Read the model definition and answer for the solid it produces. Units are mm, in the model's axes. Face numbers are marked on the shaded views. Coordinates: 2 decimals unless noted, no trailing zeros. Order: outer loops, then holes, each group sorted by start corner. A loop starts at its lowest first (then second) coordinate and runs counter-clockwise, first axis right, second up. Notation, with made-up numbers: (15.5, 26.5) -> (47.5, 26.5) arc R20 ccw to (47.5, 55.5) -> close; hole circle Ø6 at (-29, 32). An arc over 180 degrees is marked (long way). Answer as a JSON object with one key per item and string values. Group by question number.
1) Determine the mould class of the marked faces 1, 2 and 3 for opening direction Y: released by +Y, released by -Y, zero draft, split by the parting line, or undercut.
2) Section D-D on x = 6 is taken. Determine the outline of the cut face in (y, z), and give its area (3 significant figures).
3) Consider L1, parallel to X at y = -0.75, z = 101.6; L2, parallel to Y at x = 13, z = 32.5; L3, parallel to Y at x = 27.5, z = 86.5. Determine where each line is inside the solid, lowest interval first.
4) Section C-C on z = 85 is taken. Determine the outline of the cut face in (x, y) (3 decimals), and give its area (3 significant figures).
5) Section A-A on x = 29 is taken. Determine the outline of the cut face in (y, z).
6) Given pin 1 (2 mm diameter, centred on y = -16, z = 58.5, fed in from +X); pin 2 (12 mm diameter, centred on x = 17, z = 80.5, fed in from -Y); pin 3 (3 mm diameter, centred on y = -11.5, z = 48, fed in from +X), each flat-ended and moving along its own axis, determine where each tip first touches the part or whether it passes through.
7) Section B-B on z = 101.6 is taken. Determine the outline of the cut face in (x, y) (3 decimals), and give its area (3 significant figures).
from build123d import *

# Parameters (mm, degrees)
BASE_FLANGE1_DEPTH = 127
CUT_EXTRUDE1_REACH = 146.789
SKETCH6_R          = 3.175
CUT_EXTRUDE2_REACH = 139.304
SKETCH7_R          = 3.175


# Read off the part's stored shape, not the designer's step: Base-Flange1
with BuildPart() as part:
    # Base-Flange1 outline → Base-Flange1 (new body)
    with BuildSketch(Plane.XY):
        with BuildLine():
            Line((44.523372088, -7.173652981), (24.703656185, -49.677170897))
            Line((24.703656185, -49.677170897), (27.111570966, -50.8))
            Line((27.111570966, -50.8), (46.931286869, -8.296482084))
            ThreePointArc((46.931286869, -8.296482084), (46.564368833, -2.698394652), (41.645844864, 0))
            Line((41.645844864, 0), (0, 0))
            Line((0, 0), (0, -2.65684))
            Line((0, -2.65684), (41.645844864, -2.65684))
            ThreePointArc((41.645844864, -2.65684), (44.323612704, -4.125913744), (44.523372088, -7.173652981))
        make_face()
    extrude(amount=BASE_FLANGE1_DEPTH)

    # Sketch6 → Cut-Extrude1 (cut, up to next)
    with BuildSketch(Plane(origin=(0, 0, 0), x_dir=(1, 0, 0), z_dir=(0, 1, 0)), mode=Mode.PRIVATE) as cut_extrude1_sk1:
        with Locations(Location((16.245844864, -101.6, 0), (0, 0, 270))):
            Circle(SKETCH6_R)
    cut_extrude1_tool1 = extrude(cut_extrude1_sk1.sketch, amount=-CUT_EXTRUDE1_REACH, mode=Mode.PRIVATE) & part.part
    # Sketch6 → Cut-Extrude1 (cut, up to next)
    with BuildSketch(Plane(origin=(0, 0, 0), x_dir=(1, 0, 0), z_dir=(0, 1, 0)), mode=Mode.PRIVATE) as cut_extrude1_sk2:
        with Locations(Location((16.245844864, -25.4, 0), (0, 0, 270))):
            Circle(SKETCH6_R)
    cut_extrude1_tool2 = extrude(cut_extrude1_sk2.sketch, amount=-CUT_EXTRUDE1_REACH, mode=Mode.PRIVATE) & part.part
    add(cut_extrude1_tool1.solids().sort_by_distance((16.245845, 0, 101.6))[0], mode=Mode.SUBTRACT)
    add(cut_extrude1_tool2.solids().sort_by_distance((16.245845, 0, 25.4))[0], mode=Mode.SUBTRACT)

    # Sketch7 → Cut-Extrude2 (cut, up to next)
    with BuildSketch(Plane(origin=(41.726805286, -19.457528855, 0), x_dir=(0, 0, -1), z_dir=(0.906307787036648, -0.4226182617407038, 0)), mode=Mode.PRIVATE) as cut_extrude2_sk1:
        with Locations(Location((-101.6, -12.580218597, 0), (0, 0, 90))):
            Circle(SKETCH7_R)
    cut_extrude2_tool1 = extrude(cut_extrude2_sk1.sketch, amount=-CUT_EXTRUDE2_REACH, mode=Mode.PRIVATE) & part.part
    # Sketch7 → Cut-Extrude2 (cut, up to next)
    with BuildSketch(Plane(origin=(41.726805286, -19.457528855, 0), x_dir=(0, 0, -1), z_dir=(0.906307787036648, -0.4226182617407038, 0)), mode=Mode.PRIVATE) as cut_extrude2_sk2:
        with Locations(Location((-25.4, -12.580218597, 0), (0, 0, 90))):
            Circle(SKETCH7_R)
    cut_extrude2_tool2 = extrude(cut_extrude2_sk2.sketch, amount=-CUT_EXTRUDE2_REACH, mode=Mode.PRIVATE) & part.part
    add(cut_extrude2_tool1.solids().sort_by_distance((36.410175, -30.859079, 101.6))[0], mode=Mode.SUBTRACT)
    add(cut_extrude2_tool2.solids().sort_by_distance((36.410175, -30.859079, 25.4))[0], mode=Mode.SUBTRACT)


solid = part.part
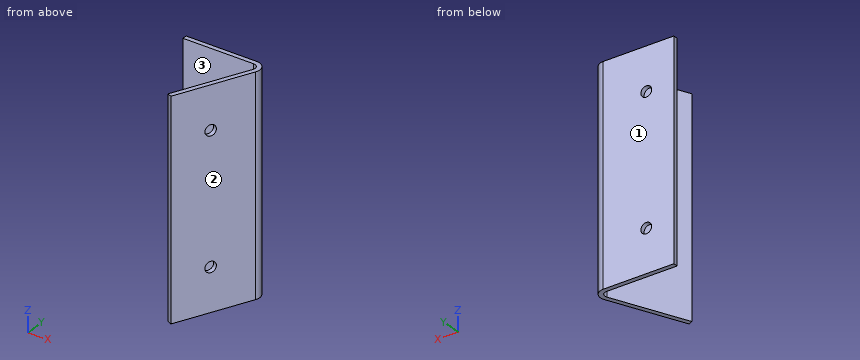
Worked answers:
{
 "1": {"face 1": "released by +Y", "face 2": "released by -Y", "face 3": "undercut"},
 "2": {"outline": "(-2.66, 0) -> (0, 0) -> (0, 127) -> (-2.66, 127) -> close", "area": "337 mm²"},
 "3": {"L1": "x = 0 to 13.07, 19.42 to 44.51", "L2": "y = -2.66 to 0", "L3": "y = -49.97 to -43.68, -2.66 to 0"},
 "4": {"outline": "(0, -2.657) -> (41.646, -2.657) arc R3.175 cw to (44.523, -7.174) -> (24.704, -49.677) -> (27.112, -50.8) -> (46.931, -8.296) arc R5.832 ccw to (41.646, 0) -> (0, 0) -> close", "area": "259 mm²"},
 "5": {"outline": "(-46.75, 0) -> (-40.46, 0) -> (-40.46, 127) -> (-46.75, 127) -> close; (-2.66, 0) -> (0, 0) -> (0, 127) -> (-2.66, 127) -> close"},
 "6": {"pin 1": "stops at x = 43.81", "pin 2": "stops at y = -2.66", "pin 3": "stops at x = 46.14"},
 "7": {"outline": "(0, -2.657) -> (13.071, -2.657) -> (13.071, 0) -> (0, 0) -> close; (19.421, -2.657) -> (41.646, -2.657) arc R3.175 cw to (44.523, -7.174) -> (35.344, -26.859) -> (37.752, -27.982) -> (46.931, -8.296) arc R5.832 ccw to (41.646, 0) -> (19.421, 0) -> close; (24.704, -49.677) -> (27.112, -50.8) -> (35.068, -33.737) -> (32.66, -32.614) -> close", "area": "226 mm²"}
}
